Input: part model. Units: mm. Frame: model coordinates. Give positions to 0.01 mm unless a question says otherwise; leave off trailing zeros. Order: outer loops, then holes, each group sorted by start corner. A loop starts at its lowest first (then second) coordinate and runs counter-clockwise, first axis right, second up. Notation, with made-up numbers: (12.5, 47.25) - (60.5, 47.25) arc R25 cw to (60.5, 59.25) - close; hole circle Ø8 at (-32, 53.5). An arc over 180 degrees is marked (long way). Answer in a Markdown table with one row per item. Add a question column.
1. Contact query for flat-ended pins moving along their axis: pin 1 (5.5 mm diameter, centred on x = 9.53, z = 10.13, fed in from +Y); pin 2 (8 mm diameter, centred on y = 21.67, z = 11, fed in from +X); pin 3 (11 mm diameter, centred on x = -2, z = 8, fed in from +Y); pin 4 (1.5 mm diameter, centred on y = 23.5, z = 8.5, fed in from +X). Output: stop coordinate, or through.
2. Section query D-D on y = -13. Return loops of the section in (x, z).
3. Section query A-A on z = 2.5. Return loops of the section in (x, y).
4. Section query C-C on x = 8.5. Return loops of the section in (y, z).
5. Ray query, line 1 (X direction, y = -13.5, z = 12.5); line 2 (X direction, y = 2, z = 13.5); line 3 (Y direction, x = -7, z = 17.5). Return the intervals inside material, ascending. Write a range as [from, to].
6. Section query B-B on x = -7. Return loops of the section in (y, z), and give its area (3 significant figures).
7. Mould query, pull axis X, two halves, no side actions, for faces 1 (the face through (-24, 33, 11)), 2 (the face through (-4, -11.326, 11)), 3 (the face through (-26.001, -5.942, 7.895)), 4 (the face through (6.117, -13.861, 10.887)). Classes: released by +X, released by -X, zero draft, split by the parting line, or undercut.
```python
from build123d import *

# Parameters (mm, degrees)
BOSS_EXTRUDE1_DEPTH = 22
FILLET1_R           = 10
FILLET2_R           = 10
SKETCH2_R           = 3.5
CUT_EXTRUDE2_DEPTH  = 50
SKETCH4_R           = 3.5
CUT_EXTRUDE3_DEPTH  = 50


with BuildPart() as part:
    # Sketch1 → Boss-Extrude1 (new body)
    with BuildSketch(Plane.XY):
        Polygon((-28.466334251, 33.673519048), (-28.466334251, -16.326480952), (21.533665749, -16.326480952), (21.533665749, -11.326480952), (-23.466334251, 33.673519048), align=None)
        Polygon((14.533665749, -11.326480952), (-23.466334251, -11.326480952), (-23.466334251, 26.673519048), align=None, mode=Mode.SUBTRACT)
    extrude(amount=BOSS_EXTRUDE1_DEPTH)

    # Fillet1
    fillet1_edges = [part.edges().sort_by_distance(p)[0] for p in [
        (-23.466334251, 33.673519048, 11),
    ]]
    fillet(fillet1_edges, radius=FILLET1_R)

    # Fillet2
    fillet2_edges = [part.edges().sort_by_distance(p)[0] for p in [
        (21.533665749, -11.326480952, 11),
    ]]
    fillet(fillet2_edges, radius=FILLET2_R)

    # Sketch2 → Cut-Extrude2 (cut)
    with BuildSketch(Plane.ZY.offset(28.466334251)):
        with Locations(Location((11, 21.673519048, 0), (0, 0, 270))):
            Circle(SKETCH2_R)
        with Locations(Location((11, -4.326480952, 0), (0, 0, 270))):
            Circle(SKETCH2_R)
    extrude(amount=-CUT_EXTRUDE2_DEPTH, mode=Mode.SUBTRACT)

    # Sketch4 → Cut-Extrude3 (cut)
    with BuildSketch(Plane.XZ.offset(16.326480952)):
        with Locations(Location((-16.466334251, 10.12780984, 0), (0, 0, 270))):
            Circle(SKETCH4_R)
        with Locations(Location((9.533665749, 10.12780984, 0), (0, 0, 270))):
            Circle(SKETCH4_R)
    extrude(amount=-CUT_EXTRUDE3_DEPTH, mode=Mode.SUBTRACT)


solid = part.part
```
Answer:
| question | item | result |
|---|---|---|
| 1 | pin 1 | passes through |
| 1 | pin 2 | stops at x = -7.46 |
| 1 | pin 3 | stops at y = 17.71 |
| 1 | pin 4 | stops at x = -12.95 |
| 2 | outline | (-28.47, 0) - (21.22, 0) - (21.22, 22) - (-28.47, 22) - close; hole circle Ø7 at (-16.47, 10.13); hole circle Ø7 at (9.53, 10.13) |
| 3 | outline | (-28.47, -16.33) - (21.53, -16.33) - (21.53, -15.47) arc R10 ccw to (18.6, -8.4) - (-20.54, 30.74) arc R10 ccw to (-27.61, 33.67) - (-28.47, 33.67) - close; hole (-23.47, -11.33) - (14.53, -11.33) - (-23.47, 26.67) - close |
| 4 | outline | (-16.33, 0) - (-11.33, 0) - (-11.33, 6.78) - (-16.33, 6.78) - close; (-16.33, 13.47) - (-11.33, 13.47) - (-11.33, 22) - (-16.33, 22) - close; (-5.29, 0) - (1.71, 0) - (1.71, 6.78) - (-5.29, 6.78) - close; (-5.29, 14.36) arc R3.5 cw to (-1.85, 13.47) - (1.71, 13.47) - (1.71, 22) - (-5.29, 22) - close |
| 5 | line 1 | x = [-28.47, -19.04], [-13.89, 6.96], [12.11, 21.34] |
| 5 | line 2 | x = [-28.47, -23.47], [1.21, 8.21] |
| 5 | line 3 | y = [-16.33, -11.33], [10.21, 17.21] |
| 6 | outline | (-16.33, 0) - (-11.33, 0) - (-11.33, 22) - (-16.33, 22) - close; (10.21, 0) - (17.21, 0) - (17.21, 22) - (10.21, 22) - close |
| 6 | area | 264 mm² |
| 7 | face 1 | released by +X |
| 7 | face 2 | undercut |
| 7 | face 3 | zero draft |
| 7 | face 4 | undercut |
